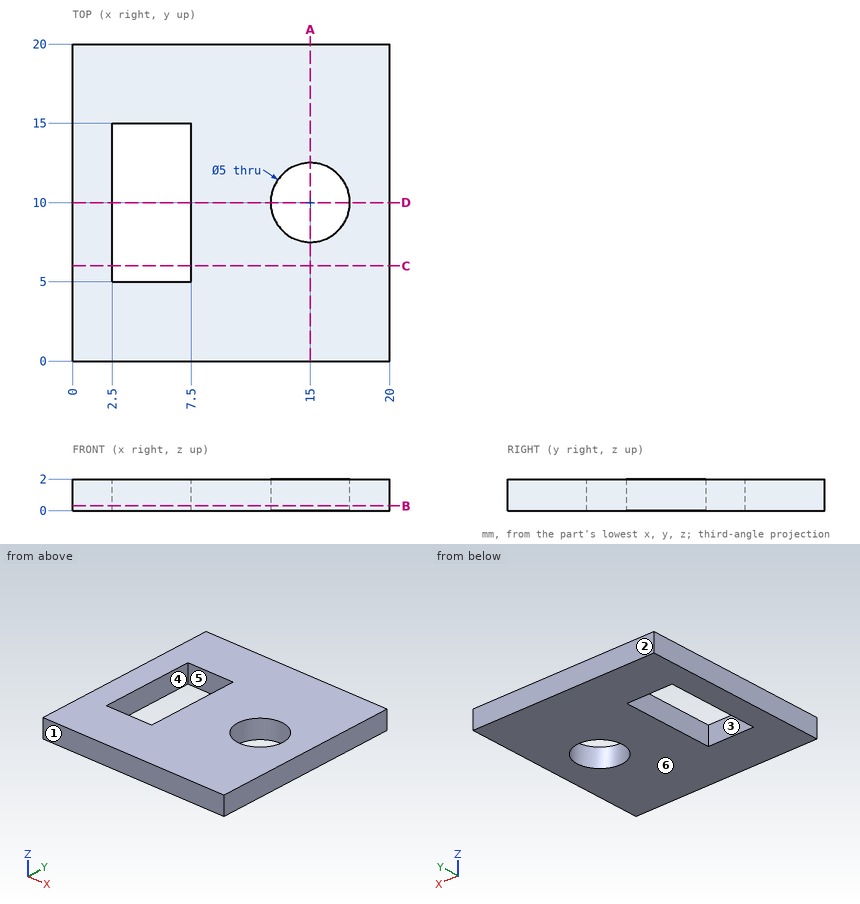
Geometry check sheet. Reference: drawing and pictorial views, mm from the part's lowest x, y, z. A direction names the side the tool comes from. Give positions to 0.01 mm unless a question says otherwise; leave off trailing zeros. Write each loop counter-clockwise with the first axis right and the second up, starting at its lowest first coordinate (ties: lowest second). Pieces come first, ordered by that corner, then holes.
Item 1: Cross-section at C-C (y = 6). Enter the section's corners in (x, z), and give its area (3 significant figures).
Item 2: Draft check along Y on the marked faces 1, 2, 3 and 4. Enter one of: released by +Y, released by -Y, zero draft, split by the parting line, or undercut.
Item 3: Access from +Z, -Z, +X, -X, +Y, -Y to the whole of each face (thin tool, end or side, straight path). Record for the marked faces 5 and 6.
Item 4: Cross-section at A-A (x = 15). Enter the section's corners in (y, z), and give its area (3 significant figures).
Item 5: Cross-section at B-B (z = 0.3). Enter the section's corners in (x, y), and give its area (3 significant figures).
Item 6: Cross-section at D-D (y = 10). Enter the section's corners in (x, z).
Item 7: Scan lines: L1, parallel to Y at x = 15, z = 0.9; L2, parallel to Y at x = 3.75, z = 0.75; L3, parallel to X at y = 14.75, z = 1.15. Record each from-to range of solid material in increasing order.
Report:
1. outline: (0, 0) - (2.5, 0) - (2.5, 2) - (0, 2) - close; (7.5, 0) - (20, 0) - (20, 2) - (7.5, 2) - close
1. area: 30.0 mm2
2. face 1: released by -Y
2. face 2: released by +Y
2. face 3: undercut
2. face 4: undercut
3. face 5: +Z, -Z
3. face 6: -Z, +X, -X, +Y, -Y
4. outline: (0, 0) - (7.5, 0) - (7.5, 2) - (0, 2) - close; (12.5, 0) - (20, 0) - (20, 2) - (12.5, 2) - close
4. area: 30.0 mm2
5. outline: (0, 0) - (20, 0) - (20, 20) - (0, 20) - close; hole (2.5, 5) - (7.5, 5) - (7.5, 15) - (2.5, 15) - close; hole circle Ø5 at (15, 10)
5. area: 330 mm2
6. outline: (0, 0) - (2.5, 0) - (2.5, 2) - (0, 2) - close; (7.5, 0) - (12.5, 0) - (12.5, 2) - (7.5, 2) - close; (17.5, 0) - (20, 0) - (20, 2) - (17.5, 2) - close
7. L1: y = 0 to 7.5, 12.5 to 20
7. L2: y = 0 to 5, 15 to 20
7. L3: x = 0 to 2.5, 7.5 to 20
